CAD build for the part. Positions are in the model's coordinates, mm. A direction names the side the tool comes from. Coordinates: 2 decimals unless noted, no trailing zeros. Write each loop counter-clockwise with the first axis right and the second up, starting at its lowest first coordinate (ties: lowest second). Pieces come first, ordered by that corner, then holes. Notation, with made-up numbers: M 63.25,-38 L 84.25,-38 A13 ccw 84.25,-17 Z; hole C 21.5,-13.75 d9. An arc over 180 degrees is marked long. Put each result on its own line as item: value. Start each with the question number.
```python
from build123d import *

# Parameters (mm, degrees)
F0_W     = 20
F0_H     = 20
F1_DEPTH = 20
F2_R     = 2.6
F3_DEPTH = 1
F4_R     = 2.6
F5_DEPTH = 1
F6_R     = 2.238333
F7_DEPTH = 1
F8_R     = 2.6
F9_DEPTH = 1
F10_R    = 1


with BuildPart() as f1:
    # F0 (on Front) → F1 (new body)
    with BuildSketch(Plane.XZ):
        with Locations((10, 10)):
            Rectangle(F0_W, F0_H)
    extrude(amount=F1_DEPTH)

    # F2 (on face) → F3 (cut)
    with BuildSketch(Plane.XZ.offset(20)):
        with Locations((10, 10)):
            Circle(F2_R)
        with Locations((5, 15)):
            Circle(F2_R)
        with Locations((15, 5)):
            Circle(F2_R)
        with Locations((15, 15)):
            Circle(F2_R)
        with Locations((5, 5)):
            Circle(F2_R)
    extrude(amount=-F3_DEPTH, mode=Mode.SUBTRACT)

    # F4 (on face) → F5 (cut)
    with BuildSketch(Plane(origin=(0, 0, 0), x_dir=(-1, 0, 0), z_dir=(0, 1, 0))):
        with Locations((-5, 15)):
            Circle(F4_R)
        with Locations((-15, 5)):
            Circle(F4_R)
    extrude(amount=-F5_DEPTH, mode=Mode.SUBTRACT)

    # F6 (on face) → F7 (cut)
    with BuildSketch(Plane.XY.offset(20)):
        with Locations((10, -10)):
            Circle(F6_R)
    extrude(amount=-F7_DEPTH, mode=Mode.SUBTRACT)

    # F8 (on face) → F9 (cut)
    with BuildSketch(Plane.YZ.offset(20)):
        with Locations((-15, 5)):
            Circle(F8_R)
        with Locations((-15, 15)):
            Circle(F8_R)
        with Locations((-5, 15)):
            Circle(F8_R)
        with Locations((-5, 5)):
            Circle(F8_R)
    extrude(amount=-F9_DEPTH, mode=Mode.SUBTRACT)

    # F10
    f10_edges = [f1.edges().sort_by_distance(p)[0] for p in [
        (20, 0, 10),
        (20, -10, 20),
        (10, 0, 20),
        (0, 0, 10),
        (0, -10, 20),
        (20, -10, 0),
        (10, 0, 0),
        (0, -10, 0),
        (0, -20, 10),
        (10, -20, 0),
        (20, -20, 10),
        (10, -20, 20),
    ]]
    fillet(f10_edges, radius=F10_R)


solid = f1.part
```
(1) Two-plate mould, pull along Z, no slides. Class faces 4 (the face through (10.126, -0.301, 19.715)), 5 (the face through (0.285, -10.126, 0.301)), 6 (the face through (0.285, -0.301, 10.126)), 7 (the face through (19, -5, 15)): +Z half, -Z half, draft (parallel to the pull), parting line (faces both ways), or undercut.
(2) Which spindle directions (+Z, -Z, +X, -X, +Y, -Y) get a long thin tool onto all of the face, cutting with end or side? Do faces 1 (the face through (19, -15, 15)), 2 (the face through (4.662, -19.507, 7.578)), 3 (the face through (10, -10, 19)). Say none if no direction does.
(3) Slice it at A-A, the plane y = -14. Write the cut outline in (x, z).
(4) Drop a flat-ended pin along its axis: pin 1 (1.6 mm diameter, centred on y = -16, z = 15.5, fed in from +X). Give the stop position or say it passes through.
(5) Drill centre lines: line 1 (Z direction, x = 5, y = -19.7); line 2 (Z direction, x = 19.3, y = -15); line 3 (Y direction, x = 13.75, z = 13.5). Where is each one in solid material? Low to high. Write a range as [from, to].
(6) Slice it at B-B, the plane z = 15. Write the cut outline in (x, y), then the cut area to 3 significant figures.
(7) Slice it at D-D, the plane y = -5. Write the cut outline in (x, z), then the cut area to 3 significant figures.
(8) Slice it at C-C, the plane x = 15. Write the cut outline in (y, z), then the cut area to 3 significant figures.
Result set:
1. face 4: +Z half
1. face 5: -Z half
1. face 6: draft
1. face 7: undercut
2. face 1: +X
2. face 2: -Y
2. face 3: +Z
3. outline: M 0,1 A1 ccw 1,0 L 19,0 A1 ccw 20,1 L 20,2.6 L 19,2.6 L 19,7.4 L 20,7.4 L 20,12.6 L 19,12.6 L 19,17.4 L 20,17.4 L 20,19 A1 ccw 19,20 L 1,20 A1 ccw 0,19 Z
4. pin 1: stops at x = 19
5. line 1: z = [0.29, 2.4], [7.6, 12.4], [17.6, 19.71]
5. line 2: z = [0.05, 2.4], [7.6, 12.4], [17.6, 19.95]
5. line 3: y = [-19, 0]
6. outline: M 0,-19 A1 ccw 1,-20 L 2.4,-20 L 2.4,-19 L 7.6,-19 L 7.6,-20 L 12.4,-20 L 12.4,-19 L 17.6,-19 L 17.6,-20 L 19,-20 A1 ccw 20,-19 L 20,-17.6 L 19,-17.6 L 19,-12.4 L 20,-12.4 L 20,-7.6 L 19,-7.6 L 19,-2.4 L 20,-2.4 L 20,-1 A1 ccw 19,0 L 7.6,0 L 7.6,-1 L 2.4,-1 L 2.4,0 L 1,0 A1 ccw 0,-1 Z
6. area: 373 mm^2
7. outline: M 0,1 A1 ccw 1,0 L 19,0 A1 ccw 20,1 L 20,2.4 L 19,2.4 L 19,7.6 L 20,7.6 L 20,12.4 L 19,12.4 L 19,17.6 L 20,17.6 L 20,19 A1 ccw 19,20 L 1,20 A1 ccw 0,19 Z
7. area: 389 mm^2
8. outline: M -20,1 A1 ccw -19,0 L -1,0 A1 ccw 0,1 L 0,2.4 L -1,2.4 L -1,7.6 L 0,7.6 L 0,19 A1 ccw -1,20 L -19,20 A1 ccw -20,19 L -20,17.6 L -19,17.6 L -19,12.4 L -20,12.4 L -20,7.6 L -19,7.6 L -19,2.4 L -20,2.4 Z
8. area: 384 mm^2
